from build123d import *

# Parameters (mm, degrees)
SKETCH1_R           = 16.15
BOSS_EXTRUDE1_DEPTH = 16.5
SKETCH2_OUTSIDE_W   = 44.014
SKETCH2_OUTSIDE_H   = 44.014
SKETCH2_OUTSIDE_R   = 13.55
CUT_EXTRUDE1_DEPTH  = 1.5
SKETCH3_R           = 9.5
CUT_EXTRUDE2_DEPTH  = 1.5
SKETCH4_OUTSIDE_W   = 44.014
SKETCH4_OUTSIDE_H   = 44.014
SKETCH4_OUTSIDE_R   = 13.55
CUT_EXTRUDE3_DEPTH  = 1.5
SKETCH5_R           = 12
CUT_EXTRUDE4_DEPTH  = 1.5
SKETCH6_R           = 1.4
CUT_EXTRUDE7_DEPTH  = 2.5
FILLET2_R           = 1.5


with BuildPart() as part:
    # Sketch1 → Boss-Extrude1 (new body)
    with BuildSketch(Plane(origin=(0, 0, 0), x_dir=(1, 0, 0), z_dir=(0, 1, 0))):
        with Locations(Location((0, 0, 0), (0, 0, 270))):
            Circle(SKETCH1_R)
    extrude(amount=-BOSS_EXTRUDE1_DEPTH)

    # Sketch2 outside → Cut-Extrude1 (cut)
    with BuildSketch(Plane(origin=(0, 0, 0), x_dir=(1, 0, 0), z_dir=(0, 1, 0))):
        Rectangle(SKETCH2_OUTSIDE_W, SKETCH2_OUTSIDE_H)
        with Locations(Location((0, 0, 0), (0, 0, 270))):
            Circle(SKETCH2_OUTSIDE_R, mode=Mode.SUBTRACT)
    extrude(amount=-CUT_EXTRUDE1_DEPTH, mode=Mode.SUBTRACT)

    # Sketch3 → Cut-Extrude2 (cut)
    with BuildSketch(Plane(origin=(0, 0, 0), x_dir=(1, 0, 0), z_dir=(0, 1, 0))):
        with Locations(Location((0, 0, 0), (0, 0, 270))):
            Circle(SKETCH3_R)
    extrude(amount=-CUT_EXTRUDE2_DEPTH, mode=Mode.SUBTRACT)

    # Sketch4 outside → Cut-Extrude3 (cut)
    with BuildSketch(Plane(origin=(0, -16.5, 0), x_dir=(-1, 0, 0), z_dir=(0, -1, 0))):
        Rectangle(SKETCH4_OUTSIDE_W, SKETCH4_OUTSIDE_H)
        with Locations(Location((0, 0, 0), (0, 0, 270))):
            Circle(SKETCH4_OUTSIDE_R, mode=Mode.SUBTRACT)
    extrude(amount=-CUT_EXTRUDE3_DEPTH, mode=Mode.SUBTRACT)

    # Sketch5 → Cut-Extrude4 (cut)
    with BuildSketch(Plane(origin=(0, -16.5, 0), x_dir=(-1, 0, 0), z_dir=(0, -1, 0))):
        with Locations(Location((0, 0, 0), (0, 0, 90))):
            Circle(SKETCH5_R)
    extrude(amount=-CUT_EXTRUDE4_DEPTH, mode=Mode.SUBTRACT)

    # Sketch6 → Cut-Extrude7 (cut)
    with BuildSketch(Plane(origin=(0, -16.5, 0), x_dir=(-1, 0, 0), z_dir=(0, -1, 0))):
        with Locations(Location((0, 8.5, 0), (0, 0, 90))):
            Circle(SKETCH6_R)
        with Locations(Location((6.01040764, 6.01040764, 0), (0, 0, 90))):
            Circle(SKETCH6_R)
        with Locations(Location((-6.01040764, 6.01040764, 0), (0, 0, 90))):
            Circle(SKETCH6_R)
        with Locations(Location((0, -8.5, 0), (0, 0, 90))):
            Circle(SKETCH6_R)
    extrude(amount=-CUT_EXTRUDE7_DEPTH, mode=Mode.SUBTRACT)

    # Fillet2
    fillet2_edges = [part.edges().sort_by_distance(p)[0] for p in [
        (0, 0, -13.55),
    ]]
    fillet(fillet2_edges, radius=FILLET2_R - 0.0001)  # a hair under: the kernel refuses the full size


solid = part.part
For this review, take the finished solid that the model builds, in its own axes (mm). A direction names the side the tool comes from. Give positions to 0.01 mm unless a question says otherwise; leave off trailing zeros. Loops run counter-clockwise (first coordinate to the right, second up) from the corner with the lowest first, then second, coordinate; pieces in that order, holes last. Notation, with made-up numbers: M -33,9 L 25,9 A22 ccw 25,27 Z; hole C -37.75,33 d4. An arc over 180 degrees is marked long. Put each result on its own line as item: value. Start each with the question number.
(1) Add section C-C, the plane y = -4.75. Write out the cut boundary in (x, z).
(2) Machinability: for faces 1 (the cylindrical face through (-15.766, -8.156, -3.501)), 2 (the flat face through (0, -15, 0)), 3 (the cylindrical face through (-5.78, -0.74, -7.54)), which of the approach directions +Z, -Z, +X, -X, +Y, -Y give a long, thin tool a straight path to every point of the face, cutting with its end or side? Answer none if there is none.
(3) The part is to be moulded in two halves that separate along X. For faces 4 (the flat face through (-3.7, -1.5, -13.2)), 5 (the cylindrical face through (4.644, -14.507, -5.707)), 6 (the cylindrical face through (5.19, -15.76, 12.517)), say which applies: +X half, -X half, draft (parallel to the pull), parting line (faces both ways), or undercut.
(4) Wall thickness on L1, parallel to Y at x = -1, z = -8.5; L2, parallel to Y at x = 1.5, z = 11; L3, parallel to X at y = -14.7, z = -8.5: over which ranges is each line inside the solid? List them lowest first.
(5) For pin 1 (3 mm diameter, centred on x = 12.5, z = 6.5, fed in from +Y); pin 2 (17 mm diameter, centred on x = 0, z = 0, fed in from -Y); pin 3 (0.8 mm diameter, centred on x = 6, z = -5.5, fed in from -Y), all flat-tipped, find the tip position at first contact; note any pin that passes through.
Result:
1. outline: C 0,0 d32.3
2. face 1: +Y, -Y
2. face 2: -Y
2. face 3: +Y
3. face 4: draft
3. face 5: undercut
3. face 6: parting line
4. L1: y = -14 to -1.5
4. L2: y = -15 to 0
4. L3: x = -13.73 to -1.4, 1.4 to 13.73
5. pin 1: stops at y = -0.1
5. pin 2: stops at y = -15
5. pin 3: stops at y = -14
